Verification items for the finished model (mm, model axes). A direction names the side the tool comes from. Give positions to 0.01 mm unless a question says otherwise; leave off trailing zeros. Write each loop counter-clockwise with the first axis right and the second up, starting at its lowest first coordinate (ties: lowest second). Pieces come first, ordered by that corner, then holes.
from build123d import *

# Parameters (mm, degrees)
BOSS_EXTRUDE1_DEPTH = 6.35
SKETCH2_R           = 2.4892
CUT_EXTRUDE1_DEPTH  = 294.699684882
SKETCH3_R           = 2.4892
CUT_EXTRUDE2_DEPTH  = 294.699684882


with BuildPart() as part:
    # Sketch1 → Boss-Extrude1 (new body)
    with BuildSketch(Plane.XY):
        with BuildLine():
            Line((12.7, 0), (241.3, 0))
            ThreePointArc((241.3, 0), (250.280256121, 3.719743879), (254, 12.7))
            Line((254, 12.7), (254, 51.507746743))
            ThreePointArc((254, 51.507746743), (252.641048665, 63.179195107), (248.636901303, 74.226197394))
            Line((248.636901303, 74.226197394), (215.600193669, 140.299612663))
            ThreePointArc((215.600193669, 140.299612663), (210.917753467, 145.423265266), (204.240968343, 147.32))
            Line((204.240968343, 147.32), (49.759031657, 147.32))
            ThreePointArc((49.759031657, 147.32), (43.082246533, 145.423265266), (38.399806331, 140.299612663))
            Line((38.399806331, 140.299612663), (5.363098697, 74.226197394))
            ThreePointArc((5.363098697, 74.226197394), (1.358951335, 63.179195107), (0, 51.507746743))
            Line((0, 51.507746743), (0, 12.7))
            ThreePointArc((0, 12.7), (3.719743879, 3.719743879), (12.7, 0))
        make_face()
        with BuildLine():
            Line((40.939806331, 81.879612663), (53.639806331, 107.279612663))
            ThreePointArc((53.639806331, 107.279612663), (58.322246533, 112.403265266), (64.999031657, 114.3))
            Line((64.999031657, 114.3), (189.000968343, 114.3))
            ThreePointArc((189.000968343, 114.3), (195.677753467, 112.403265266), (200.360193669, 107.279612663))
            Line((200.360193669, 107.279612663), (213.060193669, 81.879612663))
            ThreePointArc((213.060193669, 81.879612663), (212.504233609, 69.523214876), (201.700968343, 63.5))
            Line((201.700968343, 63.5), (52.299031657, 63.5))
            ThreePointArc((52.299031657, 63.5), (41.495766391, 69.523214876), (40.939806331, 81.879612663))
        make_face(mode=Mode.SUBTRACT)
    extrude(amount=BOSS_EXTRUDE1_DEPTH)

    # Sketch2 → Cut-Extrude1 (cut, through all)
    with BuildSketch(Plane.XY.offset(6.35)):
        with Locations((241.3, 12.7)):
            Circle(SKETCH2_R)
        with Locations((215.9, 12.7)):
            Circle(SKETCH2_R)
        with Locations((190.5, 12.7)):
            Circle(SKETCH2_R)
        with Locations((165.1, 12.7)):
            Circle(SKETCH2_R)
        with Locations((139.7, 12.7)):
            Circle(SKETCH2_R)
        with Locations((114.3, 12.7)):
            Circle(SKETCH2_R)
        with Locations((88.9, 12.7)):
            Circle(SKETCH2_R)
        with Locations((63.5, 12.7)):
            Circle(SKETCH2_R)
        with Locations((38.1, 12.7)):
            Circle(SKETCH2_R)
        with Locations((12.7, 12.7)):
            Circle(SKETCH2_R)
        with Locations((215.9, 38.1)):
            Circle(SKETCH2_R)
        with Locations((190.5, 38.1)):
            Circle(SKETCH2_R)
        with Locations((165.1, 38.1)):
            Circle(SKETCH2_R)
        with Locations((139.7, 38.1)):
            Circle(SKETCH2_R)
        with Locations((114.3, 38.1)):
            Circle(SKETCH2_R)
        with Locations((88.9, 38.1)):
            Circle(SKETCH2_R)
        with Locations((63.5, 38.1)):
            Circle(SKETCH2_R)
        with Locations((38.1, 38.1)):
            Circle(SKETCH2_R)
        with Locations((12.7, 38.1)):
            Circle(SKETCH2_R)
        with Locations((241.3, 38.1)):
            Circle(SKETCH2_R)
        with Locations((25.4, 25.4)):
            Circle(SKETCH2_R)
        with Locations((50.8, 25.4)):
            Circle(SKETCH2_R)
        with Locations((76.2, 25.4)):
            Circle(SKETCH2_R)
        with Locations((101.6, 25.4)):
            Circle(SKETCH2_R)
        with Locations((127, 25.4)):
            Circle(SKETCH2_R)
        with Locations((152.4, 25.4)):
            Circle(SKETCH2_R)
        with Locations((177.8, 25.4)):
            Circle(SKETCH2_R)
        with Locations((203.2, 25.4)):
            Circle(SKETCH2_R)
        with Locations((228.6, 25.4)):
            Circle(SKETCH2_R)
    extrude(amount=-CUT_EXTRUDE1_DEPTH, mode=Mode.SUBTRACT)

    # Sketch3 → Cut-Extrude2 (cut, through all)
    with BuildSketch(Plane.XY.offset(6.35)):
        with Locations((57.15, 130.81)):
            Circle(SKETCH3_R)
        with Locations((127, 130.81)):
            Circle(SKETCH3_R)
        with Locations((196.85, 130.81)):
            Circle(SKETCH3_R)
        with Locations((228.6, 59.332735968)):
            Circle(SKETCH3_R)
        with Locations((25.4, 59.332735968)):
            Circle(SKETCH3_R)
    extrude(amount=-CUT_EXTRUDE2_DEPTH, mode=Mode.SUBTRACT)


solid = part.part
Item 1: Sectioned sample at C-C on x = 101.6. Record the cut outline in (y, z).
Answer key:
outline: (0, 0) - (22.91, 0) - (22.91, 6.35) - (0, 6.35) - close; (27.89, 0) - (63.5, 0) - (63.5, 6.35) - (27.89, 6.35) - close; (114.3, 0) - (147.32, 0) - (147.32, 6.35) - (114.3, 6.35) - close
Item 2: Release check for a two-part mould opening along Y. For faces 3 (the face through (47, 94, 3)), 4 (the face through (125, 58, 6.35)), 5 (the face through (211, 145.37, 3.13)) record: released by +Y, released by -Y, zero draft, split by the parting line, or undercut.
Answer key:
face 3: undercut
face 4: zero draft
face 5: released by +Y
Item 3: Sectioned sample at B-B on y = 101. Record the cut outline in (x, z).
Answer key:
outline: (18.75, 0) - (50.5, 0) - (50.5, 6.35) - (18.75, 6.35) - close; (203.5, 0) - (235.25, 0) - (235.25, 6.35) - (203.5, 6.35) - close
Item 4: Sectioned sample at D-D on y = 38.1. State how many separate pieces and enclosed holes the cut face has, then the cut area to 3 significant figures.
Answer key:
separate pieces: 11
enclosed holes: 0
area: 1,300 mm2
Item 5: Set-up check for faces 1 (the face through (252.68, 63.02, 3.13)), 2 (the face through (58.24, 112.35, 3.13)): record each of +Z, -Z, +X, -X, +Y, -Y from which the full face is reachable in a straight line by a thin tool's end or side.
Answer key:
face 1: +Z, -Z, +X, +Y
face 2: +Z, -Z
Item 6: Scan lines: line 1 along Y through (x, z) = (177.8, 2); line 2 along Y through (x, z) = (139.7, 1.5); line 3 along Y through (x, z) = (155, 1.5). Record each from-to range of solid material in increasing order.
Answer key:
line 1: y = 0 to 22.91, 27.89 to 63.5, 114.3 to 147.32
line 2: y = 0 to 10.21, 15.19 to 35.61, 40.59 to 63.5, 114.3 to 147.32
line 3: y = 0 to 63.5, 114.3 to 147.32
Item 7: Depth check by flat-ended pin: pin 1 (6.5 mm diameter, centred on x = 38.1, y = 12.7, fed in from +Z); pin 2 (1 mm diameter, centred on y = 129, z = 3.5, fed in from -X). Enter the tip coordinate at first touch or a pass-through.
Answer key:
pin 1: stops at z = 6.35
pin 2: stops at x = 32.5
Item 8: Sectioned sample at A-A on x = 25.4. Record the cut outline in (y, z), then the cut area to 3 significant figures.
Answer key:
outline: (0, 0) - (22.91, 0) - (22.91, 6.35) - (0, 6.35) - close; (27.89, 0) - (56.84, 0) - (56.84, 6.35) - (27.89, 6.35) - close; (61.82, 0) - (114.3, 0) - (114.3, 6.35) - (61.82, 6.35) - close
area: 663 mm2
